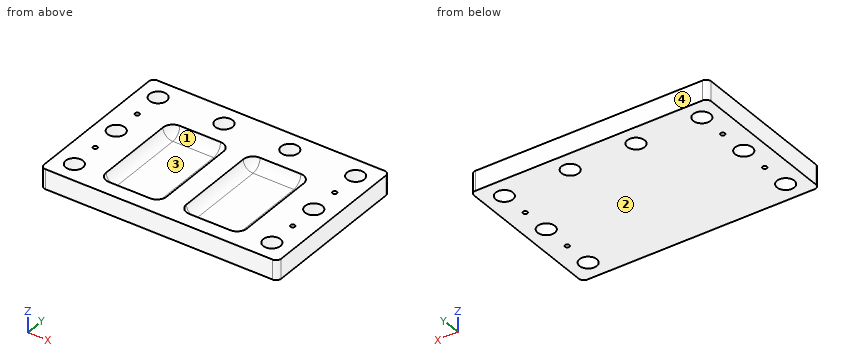
```python
from build123d import *

# Parameters (mm, degrees)
F1_DEPTH = 12.7
F3_R     = 5.55625
F4_DEPTH = 12.701
F2_R     = 1.3890625
F5_DEPTH = 12.701
F7_DEPTH = 6.35
F8_R     = 6.34999
F9_R     = 6.34999


# Not quite as in the source:
# - a fillet or chamfer is up to 0.001 mm smaller than in the source, because OpenCascade refuses the exact size


with BuildPart() as f1:
    # F0 (on Top) → F1 (new body)
    with BuildSketch(Plane.XY):
        with BuildLine():
            Line((-73.025, -50.8), (73.025, -50.8))
            ThreePointArc((73.025, -50.8), (75.2700640303, -49.8700640303), (76.2, -47.625))
            Line((76.2, -47.625), (76.2, 47.625))
            ThreePointArc((76.2, 47.625), (75.2700640303, 49.8700640303), (73.025, 50.8))
            Line((73.025, 50.8), (-73.025, 50.8))
            ThreePointArc((-73.025, 50.8), (-75.2700640303, 49.8700640303), (-76.2, 47.625))
            Line((-76.2, 47.625), (-76.2, -47.625))
            ThreePointArc((-76.2, -47.625), (-75.2700640303, -49.8700640303), (-73.025, -50.8))
        make_face()
    extrude(amount=F1_DEPTH)

    # F3 (on face) → F4 (cut, through all)
    with BuildSketch(Plane.XY.offset(12.7)):
        with Locations((-63.5, 38.1)):
            Circle(F3_R)
        with Locations((63.5, 38.1)):
            Circle(F3_R)
        with Locations((63.5, -38.1)):
            Circle(F3_R)
        with Locations((-63.5, -38.1)):
            Circle(F3_R)
        with Locations((-63.5, 0)):
            Circle(F3_R)
        with Locations((63.5, 0)):
            Circle(F3_R)
        with Locations((-21.1666666667, 38.1)):
            Circle(F3_R)
        with Locations((21.1666666667, 38.1)):
            Circle(F3_R)
    extrude(amount=-F4_DEPTH, mode=Mode.SUBTRACT)

    # F2 (on face) → F5 (cut, through all)
    with BuildSketch(Plane.XY.offset(12.7)):
        with Locations((-63.5, -19.05)):
            Circle(F2_R)
        with Locations((63.5, 19.05)):
            Circle(F2_R)
        with Locations((63.5, -19.05)):
            Circle(F2_R)
        with Locations((-63.5, 19.05)):
            Circle(F2_R)
    extrude(amount=-F5_DEPTH, mode=Mode.SUBTRACT)

    # F6 (on face) → F7 (cut)
    with BuildSketch(Plane.XY.offset(12.7)):
        with BuildLine():
            ThreePointArc((-6.35, 16.66875), (-8.2098719395, 21.1588780605), (-12.7, 23.01875))
            Line((-12.7, 23.01875), (-38.89375, 23.01875))
            ThreePointArc((-38.89375, 23.01875), (-43.3838780605, 21.1588780605), (-45.24375, 16.66875))
            Line((-45.24375, 16.66875), (-45.24375, -34.925))
            ThreePointArc((-45.24375, -34.925), (-43.3838780605, -39.4151280605), (-38.89375, -41.275))
            Line((-38.89375, -41.275), (-12.7, -41.275))
            ThreePointArc((-12.7, -41.275), (-8.2098719395, -39.4151280605), (-6.35, -34.925))
            Line((-6.35, -34.925), (-6.35, 16.66875))
        make_face()
        with BuildLine():
            ThreePointArc((6.35, -34.925), (8.2098719395, -39.4151280605), (12.7, -41.275))
            Line((12.7, -41.275), (38.89375, -41.275))
            ThreePointArc((38.89375, -41.275), (43.3838780605, -39.4151280605), (45.24375, -34.925))
            Line((45.24375, -34.925), (45.24375, 16.66875))
            ThreePointArc((45.24375, 16.66875), (43.3838780605, 21.1588780605), (38.89375, 23.01875))
            Line((38.89375, 23.01875), (12.7, 23.01875))
            ThreePointArc((12.7, 23.01875), (8.2098719395, 21.1588780605), (6.35, 16.66875))
            Line((6.35, 16.66875), (6.35, -34.925))
        make_face()
    extrude(amount=-F7_DEPTH, mode=Mode.SUBTRACT)

    # F8 (radius 6.35 in the source; OpenCascade refuses exactly that, so slightly less here)
    f8_edges = [f1.edges().sort_by_distance(p)[0] for p in [
        (-25.796875, -41.275, 6.35),
        (-6.35, -9.128125, 6.35),
        (-8.209872, -39.415128, 6.35),
        (-45.24375, -9.128125, 6.35),
        (-43.383878, -39.415128, 6.35),
        (-43.383878, 21.158878, 6.35),
        (-25.796875, 23.01875, 6.35),
        (-8.209872, 21.158878, 6.35),
    ]]
    fillet(f8_edges, radius=F8_R)

    # F9 (radius 6.35 in the source; OpenCascade refuses exactly that, so slightly less here)
    f9_edges = [f1.edges().sort_by_distance(p)[0] for p in [
        (6.35, -9.128125, 6.35),
        (8.209872, 21.158878, 6.35),
        (25.796875, 23.01875, 6.35),
        (43.383878, 21.158878, 6.35),
        (45.24375, -9.128125, 6.35),
        (43.383878, -39.415128, 6.35),
        (25.796875, -41.275, 6.35),
        (8.209872, -39.415128, 6.35),
    ]]
    fillet(f9_edges, radius=F9_R)


solid = f1.part
```
Design review of the part built by this model. Coordinates are the model's own, in mm. Face numbers are marked on the shaded views. A direction names the side the tool comes from. Give positions to 0.01 mm unless a question says otherwise; leave off trailing zeros. One line per question, with ' | ' between items. Start each with the question number.
Q1. The part is to be moulded in two halves that separate along X. For the marked faces 1 and 2, say which applies: +X half, -X half, draft (parallel to the pull), parting line (faces both ways), or undercut.
Q2. For pin 1 Ø13 at (x, y) = (21, 3) entering from +Z, flat-tipped, find the tip position at first contact; note if it passes through.
Q3. For L1, parallel to Y at x = 63.5, z = 2.5; L2, parallel to X at y = 38.5, z = 10.5; L3, parallel to X at y = 43, z = 5, list the stretches that pass through material, from the lowest coordinate up. Write a range as [from, to].
Q4. We need section A-A (y = 0). State how many separate pieces and enclosed holes the cut face has, plus the area to 3 significant figures.
Q5. Machinability: for the marked faces 3 and 4, which of the approach directions +Z, -Z, +X, -X, +Y, -Y give a long, thin tool a straight path to every point of the face, cutting with its end or side? Answer none if there is none.
Returned:
1) face 1: undercut | face 2: draft
2) pin 1: z = 6.35
3) L1: [-50.8, -43.66], [-32.54, -20.44], [-17.66, -5.56], [5.56, 17.66], [20.44, 32.54], [43.66, 50.8] | L2: [-76.2, -69.04], [-57.96, -26.71], [-15.62, 15.62], [26.71, 57.96], [69.04, 76.2] | L3: [-76.2, -66.12], [-60.88, -23.79], [-18.55, 18.55], [23.79, 60.88], [66.12, 76.2]
4) separate pieces: 3 | enclosed holes: 0 | area: 1,190 mm2
5) face 3: +Z | face 4: +Z, -Z, +X, -X, +Y
